```python
from build123d import *

# Parameters (mm, degrees)
SKETCH_1_W      = 10
SKETCH_1_H      = 20
EXTRUDE_1_DEPTH = 10
FILLET_1_R      = 7


with BuildPart() as part:
    # 草图1 → 凸台-拉伸1 (new body)
    with BuildSketch(Plane.XY):
        with Locations((-35, -30)):
            Rectangle(SKETCH_1_W, SKETCH_1_H)
    extrude(amount=EXTRUDE_1_DEPTH)

    # 圆角1
    fillet_1_edges = [part.edges().sort_by_distance(p)[0] for p in [
        (-35, -40, 10),
    ]]
    fillet(fillet_1_edges, radius=FILLET_1_R)


solid = part.part
```
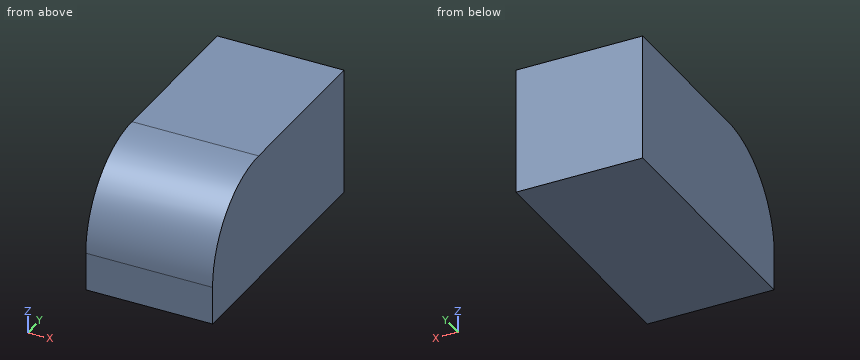
Verification items for the finished model (mm, model axes). Coordinates: 2 decimals unless noted, no trailing zeros. Write each loop counter-clockwise with the first axis right and the second up, starting at its lowest first coordinate (ties: lowest second). Pieces come first, ordered by that corner, then holes. Notation, with made-up numbers: M 39.25,-36 L 63.25,-36 A5 cw 63.25,-31 Z; hole C 48,87.5 d11. An arc over 180 degrees is marked long. Answer as a JSON object with one key per item and string values. Group by question number.
(1) Material ranges on line 1 (Z direction, x = -33.5, y = -34.25); line 2 (Y direction, x = -32.75, z = 3.5); line 3 (Y direction, x = -37.5, z = 9.25), recorded low to high.
(2) Cross-section at B-B, the plane z = 7. Record the cut outline in (x, y), and give its area (3 significant figures).
(3) Cross-section at A-A, the plane x = -31. Record the cut outline in (y, z), and give its area (3 significant figures).
(4) Gauge pin test, flat end, axial feed: pin 1 (6 mm diameter, centred on x = -32.5, y = -25.5, fed in from -Z). Record the tip position at first contact, or that the pin passes through.
(5) Cross-section at C-C, the plane y = -39. Record the cut outline in (x, z).
Reply:
{
 "1": {"line 1": "0 to 9.89", "line 2": "-39.98 to -20", "line 3": "-36.15 to -20"},
 "2": {"outline": "M -40,-38.74 L -30,-38.74 L -30,-20 L -40,-20 Z", "area": "187 mm²"},
 "3": {"outline": "M -40,0 L -20,0 L -20,10 L -33,10 A7 ccw -40,3 Z", "area": "189 mm²"},
 "4": {"pin 1": "z = 0"},
 "5": {"outline": "M -40,0 L -30,0 L -30,6.61 L -40,6.61 Z"}
}
